Geometry check sheet. Reference: the model listing, model coordinates, mm. Give positions to 0.01 mm unless a question says otherwise; leave off trailing zeros. Loops run counter-clockwise (first coordinate to the right, second up) from the corner with the lowest first, then second, coordinate; pieces in that order, holes last. Notation, with made-up numbers: (9, -7.75) -> (21, -7.75) arc R11 cw to (21, 1.25) -> close; hole circle Ø1 at (33.5, 24.25). An arc over 180 degrees is marked (long way). One line per question, with ' | ' between items.
from build123d import *

# Parameters (mm, degrees)
SKETCH2_R           = 100
SKETCH2_R_2         = 1.49
SKETCH2_R_3         = 1.7
BOSS_EXTRUDE1_DEPTH = 4
SKETCH3_R           = 1.7
CUT_EXTRUDE1_DEPTH  = 10
CUT_EXTRUDE2_START  = -4
SKETCH4_R           = 3.5
CUT_EXTRUDE2_DEPTH  = 2.5
SKETCH5_R           = 3.5
CUT_EXTRUDE3_DEPTH  = 2.5


with BuildPart() as part:
    # Sketch2 → Boss-Extrude1 (new body)
    with BuildSketch(Plane(origin=(0, 0, 0), x_dir=(1, 0, 0), z_dir=(0, 1, 0))):
        with Locations(Location((0, 0, 0), (0, 0, 270))):
            Circle(SKETCH2_R)
        with Locations(Location((59.149482246, -68.129738367, 0), (0, 0, 270))):
            Circle(SKETCH2_R_2, mode=Mode.SUBTRACT)
        with Locations(Location((68.129738367, -59.149482246, 0), (0, 0, 270))):
            Circle(SKETCH2_R_2, mode=Mode.SUBTRACT)
        with Locations(Location((-59.149482246, 68.129738367, 0), (0, 0, 270))):
            Circle(SKETCH2_R_2, mode=Mode.SUBTRACT)
        with Locations(Location((-68.129738367, 59.149482246, 0), (0, 0, 270))):
            Circle(SKETCH2_R_2, mode=Mode.SUBTRACT)
        with Locations(Location((-59.149482246, -68.129738367, 0), (0, 0, 270))):
            Circle(SKETCH2_R_2, mode=Mode.SUBTRACT)
        with Locations(Location((-68.129738367, -59.149482246, 0), (0, 0, 270))):
            Circle(SKETCH2_R_2, mode=Mode.SUBTRACT)
        with Locations(Location((68.129738367, 59.149482246, 0), (0, 0, 270))):
            Circle(SKETCH2_R_2, mode=Mode.SUBTRACT)
        with Locations(Location((59.149482246, 68.129738367, 0), (0, 0, 270))):
            Circle(SKETCH2_R_2, mode=Mode.SUBTRACT)
        with Locations(Location((-89.175, 0, 0), (0, 0, 270))):
            Circle(SKETCH2_R_3, mode=Mode.SUBTRACT)
        with Locations(Location((89.175, 0, 0), (0, 0, 270))):
            Circle(SKETCH2_R_3, mode=Mode.SUBTRACT)
    extrude(amount=BOSS_EXTRUDE1_DEPTH)

    # Sketch3 → Cut-Extrude1 (cut)
    with BuildSketch(Plane(origin=(0, 4, 0), x_dir=(1, 0, 0), z_dir=(0, 1, 0))):
        with Locations(Location((-31.993836737, 24.922768925, 0), (0, 0, 270))):
            Circle(SKETCH3_R)
        with Locations(Location((-85.380398716, -28.463793055, 0), (0, 0, 270))):
            Circle(SKETCH3_R)
        with Locations(Location((28.463793055, 85.380398716, 0), (0, 0, 270))):
            Circle(SKETCH3_R)
        with Locations(Location((-24.922768925, 31.993836737, 0), (0, 0, 270))):
            Circle(SKETCH3_R)
        with Locations(Location((31.993836737, -24.922768925, 0), (0, 0, 270))):
            Circle(SKETCH3_R)
        with Locations(Location((85.380398716, 28.463793055, 0), (0, 0, 270))):
            Circle(SKETCH3_R)
        with Locations(Location((24.922768925, -31.993836737, 0), (0, 0, 270))):
            Circle(SKETCH3_R)
        with Locations(Location((-28.463793055, -85.380398716, 0), (0, 0, 270))):
            Circle(SKETCH3_R)
    extrude(amount=-CUT_EXTRUDE1_DEPTH, mode=Mode.SUBTRACT)

    # Sketch4 → Cut-Extrude2 (cut)
    with BuildSketch(Plane(origin=(0, 4, 0), x_dir=(1, 0, 0), z_dir=(0, 1, 0)).offset(CUT_EXTRUDE2_START)):
        with Locations(Location((-85.380398716, -28.463793055, 0), (0, 0, 270))):
            Circle(SKETCH4_R)
        with Locations(Location((-68.129738367, -59.149482246, 0), (0, 0, 270))):
            Circle(SKETCH4_R)
        with Locations(Location((-59.149482246, -68.129738367, 0), (0, 0, 270))):
            Circle(SKETCH4_R)
        with Locations(Location((-28.463793055, -85.380398716, 0), (0, 0, 270))):
            Circle(SKETCH4_R)
        with Locations(Location((59.149482246, -68.129738367, 0), (0, 0, 270))):
            Circle(SKETCH4_R)
        with Locations(Location((68.129738367, -59.149482246, 0), (0, 0, 270))):
            Circle(SKETCH4_R)
        with Locations(Location((85.380398716, 28.463793055, 0), (0, 0, 270))):
            Circle(SKETCH4_R)
        with Locations(Location((68.129738367, 59.149482246, 0), (0, 0, 270))):
            Circle(SKETCH4_R)
        with Locations(Location((59.149482246, 68.129738367, 0), (0, 0, 270))):
            Circle(SKETCH4_R)
        with Locations(Location((28.463793055, 85.380398716, 0), (0, 0, 270))):
            Circle(SKETCH4_R)
        with Locations(Location((-59.149482246, 68.129738367, 0), (0, 0, 270))):
            Circle(SKETCH4_R)
        with Locations(Location((-68.129738367, 59.149482246, 0), (0, 0, 270))):
            Circle(SKETCH4_R)
        with Locations(Location((-24.922768925, 31.993836737, 0), (0, 0, 270))):
            Circle(SKETCH4_R)
        with Locations(Location((-31.993836737, 24.922768925, 0), (0, 0, 270))):
            Circle(SKETCH4_R)
        with Locations(Location((31.993836737, -24.922768925, 0), (0, 0, 270))):
            Circle(SKETCH4_R)
        with Locations(Location((24.922768925, -31.993836737, 0), (0, 0, 270))):
            Circle(SKETCH4_R)
    extrude(amount=CUT_EXTRUDE2_DEPTH, mode=Mode.SUBTRACT)

    # Sketch5 → Cut-Extrude3 (cut)
    with BuildSketch(Plane(origin=(0, 4, 0), x_dir=(1, 0, 0), z_dir=(0, 1, 0))):
        with Locations(Location((-89.175, 0, 0), (0, 0, 270))):
            Circle(SKETCH5_R)
        with Locations(Location((89.175, 0, 0), (0, 0, 270))):
            Circle(SKETCH5_R)
    extrude(amount=-CUT_EXTRUDE3_DEPTH, mode=Mode.SUBTRACT)


solid = part.part
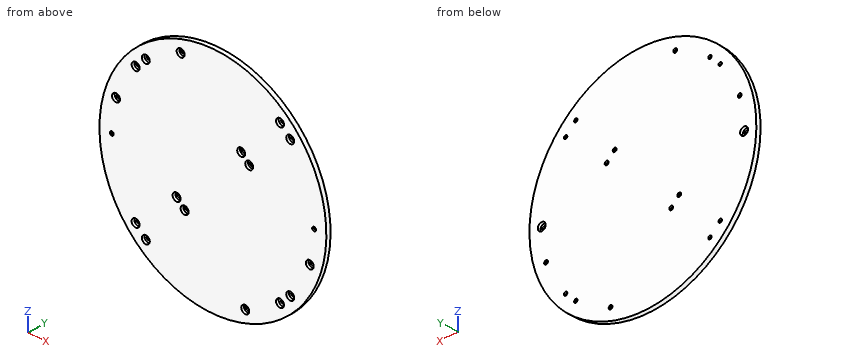
Item 1: Sectioned sample at B-B (z = 40.5). Record the cut outline in (x, y).
Result:
outline: (-91.43, 0) -> (91.43, 0) -> (91.43, 4) -> (-91.43, 4) -> close
Item 2: Depth check by flat-ended pin: pin 1 Ø3.5 at (x, z) = (60.5, 68.5) entering from -Y; pin 2 Ø2 at (x, y) = (1.5, 2.5) entering from +Z; pin 3 Ø4 at (x, z) = (89.175, 0) entering from +Y. Enter the tip coordinate at first touch or a pass-through.
Result:
pin 1: y = 2.5 | pin 2: z = 100 | pin 3: y = 1.5
Item 3: Sectioned sample at A-A (x = 45.5). Record the cut outline in (y, z).
Result:
outline: (0, -89.05) -> (4, -89.05) -> (4, 89.05) -> (0, 89.05) -> close
Item 4: Scan lines: probe 1 along X at (y, z) = (1.6, 30.5); probe 2 along Z at (x, y) = (26, 0.3); probe 3 along Z at (x, y) = (58, 1.1). Record each from-to range of solid material in increasing order.
Result:
probe 1: -95.24 to -88.23, -82.53 to 21.76, 28.09 to 95.24 | probe 2: -96.56 to -87.87, -82.89 to 28.66, 35.32 to 96.56 | probe 3: -81.46 to -71.44, -64.82 to 64.82, 71.44 to 81.46
